Read the model definition and answer for the solid it produces. Units are mm, in the model's axes. Face numbers are marked on the shaded views. A direction names the side the tool comes from. Coordinates: 2 decimals unless noted, no trailing zeros. Order: outer loops, then holes, each group sorted by start corner. A loop starts at its lowest first (then second) coordinate and runs counter-clockwise, first axis right, second up. Notation, with made-up numbers: (68.5, 54.5) - (126.5, 54.5) arc R26 cw to (126.5, 92.5) - close; hole circle Ø11 at (7.25, 35.5). An arc over 180 degrees is marked (long way). Use one line per item in the form item = value.
```python
from build123d import *

# Parameters (mm, degrees)
SKETCH1_R                    = 6.35
BOSS_EXTRUDE1_DEPTH          = 10.16
F_1_8_0_125_DIAMETER_HOLE1_D = 3.175
SKETCH4_R                    = 3.175
CUT_EXTRUDE1_DEPTH           = 5.08
CUT_EXTRUDE2_DEPTH           = 5.08
F_2_56_TAPPED_HOLE1_REACH    = 18.12
F_2_56_TAPPED_HOLE1_BORE_R   = 0.889


with BuildPart() as part:
    # Sketch1 → Boss-Extrude1 (new body)
    with BuildSketch(Plane(origin=(0, 0, 0), x_dir=(1, 0, 0), z_dir=(0, 1, 0))):
        with Locations(Location((0, 0, 0), (0, 0, 270))):
            Circle(SKETCH1_R)
    extrude(amount=BOSS_EXTRUDE1_DEPTH)

    # 1/8 (0.125) Diameter Hole1 (through all)
    with Locations(Plane(origin=(0, 10.16, 0), x_dir=(1, 0, 0), z_dir=(0, 1, 0))):
        with Locations((0, 0)):
            Hole(F_1_8_0_125_DIAMETER_HOLE1_D / 2)

    # Sketch4 → Cut-Extrude1 (cut)
    with BuildSketch(Plane(origin=(0, 10.16, 0), x_dir=(1, 0, 0), z_dir=(0, 1, 0))):
        with Locations(Location((0, 0, 0), (0, 0, 270))):
            Circle(SKETCH4_R)
    extrude(amount=-CUT_EXTRUDE1_DEPTH, mode=Mode.SUBTRACT)

    # Sketch5 → Cut-Extrude2 (cut)
    with BuildSketch(Plane(origin=(0, 10.16, 0), x_dir=(1, 0, 0), z_dir=(0, 1, 0))):
        Polygon((0, 0), (-7.62, -13.198227154), (-7.62, 13.198227154), align=None)
    cut_extrude2 = extrude(amount=-CUT_EXTRUDE2_DEPTH, mode=Mode.SUBTRACT)

    # Mirror1: Cut-Extrude2 across plane
    add(cut_extrude2.mirror(Plane(origin=(0, 0, 0), x_dir=(0, 0, 1), z_dir=(1, 0, 0))), mode=Mode.SUBTRACT)

    # #2-56 Tapped Hole1 bore (on position points) → #2-56 Tapped Hole1 (cut, up to next)
    with BuildSketch(Plane(origin=(-6.349986105, 2.54, 0.013284072), x_dir=(-0.002091979827, 0, -0.999997811808), z_dir=(-0.999997811808, 0, 0.002091979827)), mode=Mode.PRIVATE) as f_2_56_tapped_hole1_sk1:
        Circle(F_2_56_TAPPED_HOLE1_BORE_R)
    f_2_56_tapped_hole1_tool1 = extrude(f_2_56_tapped_hole1_sk1.sketch, amount=-F_2_56_TAPPED_HOLE1_REACH, mode=Mode.PRIVATE) & part.part
    add(f_2_56_tapped_hole1_tool1.solids().sort_by_distance((-6.349986, 2.54, 0.013284))[0], mode=Mode.SUBTRACT)


solid = part.part
```
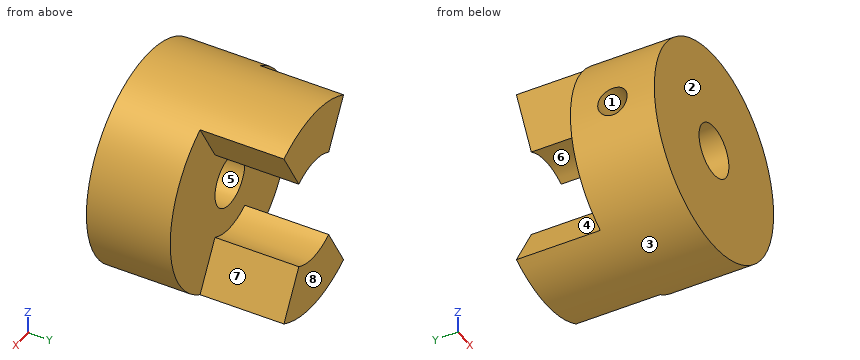
(1) Section C-C, the plane z = -5 is taken. Write down the section's boundary in (x, y), then the cut area to 3 significant figures.
Answer list:
outline = (-3.91, 0) - (3.91, 0) - (3.91, 5.08) - (2.89, 5.08) - (2.89, 10.16) - (-2.89, 10.16) - (-2.89, 5.08) - (-3.91, 5.08) - close
area = 69.1 mm2
(2) Straight lines are drawn through the part: L1, parallel to X at y = 1.4, z = 0; L2, parallel to Y at x = -4.25, z = -1. For each, find the intervals that lie inside material, in ascending order.
Answer list:
L1 = -6.35 to -1.59, 1.59 to 6.35
L2 = 0 to 5.08
(3) Given pin 1 Ø1 at (x, z) = (-5, 3.5) entering from -Y; pin 2 Ø1.5 at (x, y) = (1, 6.5) entering from +Z; pin 3 Ø1 at (x, z) = (4.5, 4) entering from +Y; pin 4 Ø1 at (x, y) = (2, 9) entering from -Z, each flat-ended and moving along its own axis, determine where each tip first touches the part or whether it passes through.
Answer list:
pin_1 = 0
pin_2 = 6.35
pin_3 = 5.08
pin_4 = -6.17
(4) Which of the six approach directions +Z, -Z, +X, -X, +Y, -Y give full straight-line access (tool end or side, diameter ignored) to the marked faces 4, 5, 6, 7 and 8?
Answer list:
face_4 = -X, +Y
face_5 = +Y, -Y
face_6 = +Y
face_7 = +X, +Y
face_8 = +Z, -Z, +X, -X, +Y
(5) The mould has two halves that part along Z. Classify the marked faces 1, 2 and 3: +Z half, -Z half, draft (parallel to the pull), parting line (faces both ways), or undercut.
Answer list:
face_1 = undercut
face_2 = draft
face_3 = parting line
